from build123d import *

# Parameters (mm, degrees)
PAD_DEPTH    = 10
FILLET_R     = 1
FILLET001_R  = 1
FILLET002_R  = 1
FILLET003_R  = 1
FILLET004_R  = 1
FILLET005_R  = 1
SKETCH001_R  = 3
POCKET_DEPTH = 5


with BuildPart() as part:
    # Sketch → Pad (new body)
    with BuildSketch(Plane.XY):
        Polygon((20, 70), (20, 10), (10, 10), (10, 80), (60, 80), (60, 10), (50, 10), (50, 70), align=None)
    extrude(amount=PAD_DEPTH)

    # Fillet
    fillet_edges = [part.edges().sort_by_distance(p)[0] for p in [
        (35, 80, 10),
    ]]
    fillet(fillet_edges, radius=FILLET_R)

    # Fillet001
    fillet001_edges = [part.edges().sort_by_distance(p)[0] for p in [
        (60, 44.5, 10),
    ]]
    fillet(fillet001_edges, radius=FILLET001_R)

    # Fillet002
    fillet002_edges = [part.edges().sort_by_distance(p)[0] for p in [
        (10, 44.5, 10),
    ]]
    fillet(fillet002_edges, radius=FILLET002_R)

    # Fillet003
    fillet003_edges = [part.edges().sort_by_distance(p)[0] for p in [
        (10, 44.5, 0),
    ]]
    fillet(fillet003_edges, radius=FILLET003_R)

    # Fillet004
    fillet004_edges = [part.edges().sort_by_distance(p)[0] for p in [
        (20, 70, 5),
    ]]
    fillet(fillet004_edges, radius=FILLET004_R)

    # Fillet005
    fillet005_edges = [part.edges().sort_by_distance(p)[0] for p in [
        (50, 70, 5),
    ]]
    fillet(fillet005_edges, radius=FILLET005_R)

    # Sketch001 (on Face8 of Fillet005) → Pocket (cut)
    with BuildSketch(Plane.XZ.offset(-10)):
        with Locations((15, 5)):
            Circle(SKETCH001_R)
        with Locations((55, 5)):
            Circle(SKETCH001_R)
    extrude(amount=-POCKET_DEPTH, mode=Mode.SUBTRACT)


solid = part.part
Can you work these out from the model? Positions are in its coordinate system, mm. A direction names the side the tool comes from. Give positions to 0.01 mm unless a question says otherwise; leave off trailing zeros. Loops run counter-clockwise (first coordinate to the right, second up) from the corner with the lowest first, then second, coordinate; pieces in that order, holes last. Notation, with made-up numbers: (-8, 57.5) -> (4, 57.5) arc R6 cw to (4, 62.5) -> close; hole circle Ø4 at (53.5, 0.5). An arc over 180 degrees is marked (long way). Write item = value, one per line.
1) I need wall thicknesses on L1, parallel to X at y = 61, z = 5.25; L2, parallel to Z at x = 15, y = 11; L3, parallel to Y at x = 38, z = 7.75. Which ranges of each line are inside material? Lowest first, please. Write a range as from..to.
Check result:
L1 = 10..20, 50..60
L2 = 0..2, 8..10
L3 = 70..80
2) Thinking about a two-plate mould opening in X: for faces 4 (the flat face through (60, 45, 5)), 5 (the flat face through (55, 15, 5)), 6 (the flat face through (35, 80, 5)), which applies, released by +X, released by -X, zero draft, split by the parting line, or undercut?
Check result:
face_4 = released by +X
face_5 = undercut
face_6 = zero draft
3) Suppose I cut it at C-C on z = 5. Write out the boundary of the cut face in (x, y).
Check result:
outline = (10, 10) -> (12, 10) -> (12, 15) -> (18, 15) -> (18, 10) -> (20, 10) -> (20, 69) arc R1 cw to (21, 70) -> (49, 70) arc R1 cw to (50, 69) -> (50, 10) -> (52, 10) -> (52, 15) -> (58, 15) -> (58, 10) -> (60, 10) -> (60, 79) arc R1 ccw to (59, 80) -> (11, 80) arc R1 ccw to (10, 79) -> close
4) For faces 1 (the cylindrical face through (52, 12, 5)), 2 (the flat face through (35, 70, 5)), 3 (the flat face through (10, 44, 5)), which set-ups out of +Z, -Z, +X, -X, +Y, -Y let a thin tool reach every point of the face, with its end or its side?
Check result:
face_1 = -Y
face_2 = +Z, -Z, -Y
face_3 = +Z, -Z, -X, +Y, -Y
5) Suppose I cut it at A-A on y = 33. Write out the boundary of the cut face in (x, z), then the cut area to 3 significant figures.
Check result:
outline = (10, 1) arc R1 ccw to (11, 0) -> (20, 0) -> (20, 10) -> (11, 10) arc R1 ccw to (10, 9) -> close; (50, 0) -> (59, 0) arc R1 ccw to (60, 1) -> (60, 9) arc R1 ccw to (59, 10) -> (50, 10) -> close
area = 199 mm2
6) Will these pins go through, and if not, where does the flat tip stop? pin 1 (5 mm diameter, centred on x = 16, z = 6, fed in from -Y); pin 2 (8 mm diameter, centred on x = 25, y = 38.5, fed in from +Z); pin 3 (2 mm diameter, centred on x = 26.5, z = 7.5, fed in from -Y); pin 4 (3 mm diameter, centred on x = 55.5, z = 5, fed in from -Y).
Check result:
pin_1 = 10
pin_2 = through
pin_3 = 70
pin_4 = 15
7) Suppose I cut it at B-B on x = 22.5. Write out the boundary of the cut face in (y, z).
Check result:
outline = (70, 0) -> (79, 0) arc R1 ccw to (80, 1) -> (80, 9) arc R1 ccw to (79, 10) -> (70, 10) -> close
8) Suppose I cut it at D-D on x = 15. Write out the boundary of the cut face in (y, z).
Check result:
outline = (10, 0) -> (79, 0) arc R1 ccw to (80, 1) -> (80, 9) arc R1 ccw to (79, 10) -> (10, 10) -> (10, 8) -> (15, 8) -> (15, 2) -> (10, 2) -> close
